Here's how the part is built. I have some questions about the finished solid (model axes, mm). Face numbers are marked on the shaded views. A direction names the side the tool comes from. Coordinates: 2 decimals unless noted, no trailing zeros. Order: outer loops, then holes, each group sorted by start corner. A loop starts at its lowest first (then second) coordinate and runs counter-clockwise, first axis right, second up. Notation, with made-up numbers: (-9, 45.25) -> (10, 45.25) arc R17 ccw to (10, 66.25) -> close; hole circle Ø7 at (59, -30). An arc over 180 degrees is marked (long way). One line per item, written item: value. Start each with the question number.
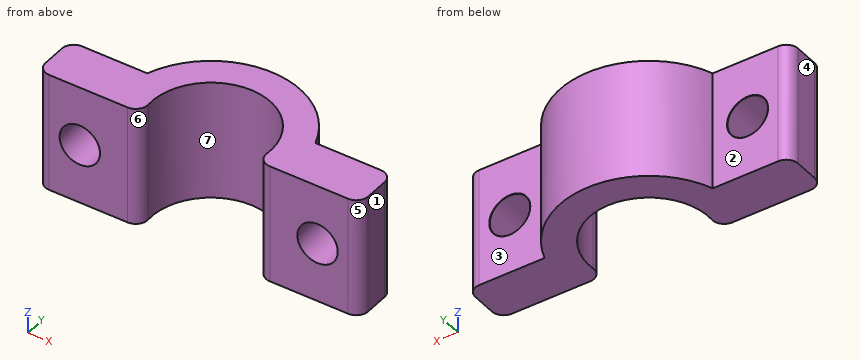
```python
from build123d import *

# Parameters (mm, degrees)
BOSS_EXTRUDE1_DEPTH            = 10
M3_CLEARANCE_HOLE1_D           = 3.4
M3_CLEARANCE_HOLE1_CSINK_D     = 3.45
M3_CLEARANCE_HOLE1_CSINK_ANGLE = 90
FILLET1_R                      = 1


with BuildPart() as part:
    # Sketch2 → Boss-Extrude1 (new body)
    with BuildSketch(Plane.XY):
        with BuildLine():
            Line((4.769696007, -1.5), (13.571067812, -1.5))
            Line((13.571067812, -1.5), (13.571067812, 2.5))
            Line((13.571067812, 2.5), (7.071067812, 2.5))
            ThreePointArc((7.071067812, 2.5), (0, 7.5), (-7.071067812, 2.5))
            Line((-7.071067812, 2.5), (-13.571067812, 2.5))
            Line((-13.571067812, 2.5), (-13.571067812, -1.5))
            Line((-13.571067812, -1.5), (-4.769696007, -1.5))
            ThreePointArc((-4.769696007, -1.5), (0, 5), (4.769696007, -1.5))
        make_face()
    extrude(amount=BOSS_EXTRUDE1_DEPTH)

    # M3 Clearance Hole1 (through all)
    with Locations(Plane(origin=(0, 2.5, 0), x_dir=(1, 0, 0), z_dir=(0, 1, 0))):
        with Locations((-10, -5), (10, -5)):
            CounterSinkHole(M3_CLEARANCE_HOLE1_D / 2, M3_CLEARANCE_HOLE1_CSINK_D / 2, counter_sink_angle=M3_CLEARANCE_HOLE1_CSINK_ANGLE)

    # Fillet1
    fillet1_edges = [part.edges().sort_by_distance(p)[0] for p in [
        (13.571067812, 2.5, 5),
        (13.571067812, -1.5, 5),
        (4.769696007, -1.5, 5),
        (-4.769696007, -1.5, 5),
        (-13.571067812, -1.5, 5),
        (-13.571067812, 2.5, 5),
    ]]
    fillet(fillet1_edges, radius=FILLET1_R)


solid = part.part
```
Q1. For P1, Ø5, axis at x = -9, z = 8.5, coming from the +Y side; P2, Ø1, axis at y = 6, z = 8, coming from the +X side; P3, Ø3, axis at x = 7, y = 3, coming from the -Z side; P4, Ø4.5, axis at x = -10.5, z = 7, coming from the +Y side, each with a flat end and sliding along its axis, tell me the tip position at first contact or that it passes through.
Q2. Imagine slicing it at A-A (y = 0). Write out the boundary of the cut face in (x, z), plus the area to 3 significant figures.
Q3. Imagine slicing it at C-C (z = 5). Write out the boundary of the cut face in (x, y) (3 decimals).
Q4. If we mould it in two halves opening along X, with no side actions, what happens to the marked faces 4, 5, 6 and 7? For each: +X half, -X half, draft (parallel to the pull), parting line (faces both ways), or undercut.
Q5. Imagine slicing it at D-D (y = 4). Write out the boundary of the cut face in (x, z).
Q6. For the marked faces 1, 2 and 3, which set-ups out of +Z, -Z, +X, -X, +Y, -Y let a thin tool reach every point of the face, with its end or its side?
Q7. I need wall thicknesses on line 1 (X direction, y = -0.1, z = 5); line 2 (X direction, y = -0.25, z = 2); line 3 (Z direction, x = 10, y = 0.45). Which ranges of each line are inside material? Lowest first, please.
Q8. Imagine slicing it at B-B (x = 10). Write out the boundary of the cut face in (y, z) (3 decimals).
Completed:
1. P1: stops at y = 3.74
1. P2: stops at x = 5.1
1. P3: stops at z = 0
1. P4: stops at y = 2.5
2. outline: (-13.57, 0) -> (-5, 0) -> (-5, 10) -> (-13.57, 10) -> close; (5, 0) -> (13.57, 0) -> (13.57, 10) -> (5, 10) -> close; hole circle Ø3.4 at (-10, 5); hole circle Ø3.4 at (10, 5)
2. area: 153 mm2
3. outline: (-13.571, -0.5) arc R1 ccw to (-12.571, -1.5) -> (-11.7, -1.5) -> (-11.7, 2.475) -> (-11.725, 2.5) -> (-12.571, 2.5) arc R1 ccw to (-13.571, 1.5) -> close; (-8.3, -1.5) -> (-5.979, -1.5) arc R1 ccw to (-4.983, -0.417) arc R5 cw (long way) to (4.983, -0.417) arc R1 ccw to (5.979, -1.5) -> (8.3, -1.5) -> (8.3, 2.475) -> (8.275, 2.5) -> (7.071, 2.5) arc R7.5 ccw to (-7.071, 2.5) -> (-8.275, 2.5) -> (-8.3, 2.475) -> close; (11.7, -1.5) -> (12.571, -1.5) arc R1 ccw to (13.571, -0.5) -> (13.571, 1.5) arc R1 ccw to (12.571, 2.5) -> (11.725, 2.5) -> (11.7, 2.475) -> close
4. face 4: -X half
4. face 5: +X half
4. face 6: undercut
4. face 7: undercut
5. outline: (-6.34, 0) -> (-3, 0) -> (-3, 10) -> (-6.34, 10) -> close; (3, 0) -> (6.34, 0) -> (6.34, 10) -> (3, 10) -> close
6. face 1: +Z, -Z, +X, +Y, -Y
6. face 2: +Z, -Z, -X, +Y
6. face 3: +Z, -Z, +X, +Y
7. line 1: x = -13.57 to -11.7, -8.3 to -5, 5 to 8.3, 11.7 to 13.57
7. line 2: x = -13.57 to -4.99, 4.99 to 13.57
7. line 3: z = 0 to 3.3, 6.7 to 10
8. outline: (-1.5, 0) -> (2.5, 0) -> (2.5, 3.275) -> (2.475, 3.3) -> (-1.5, 3.3) -> close; (-1.5, 6.7) -> (2.475, 6.7) -> (2.5, 6.725) -> (2.5, 10) -> (-1.5, 10) -> close
